```python
from build123d import *

# Parameters (mm, degrees)
SKETCH1_R           = 20
BOSS_EXTRUDE1_DEPTH = 32
SKETCH2_R           = 3
CUT_EXTRUDE1_DEPTH  = 32
CUT_EXTRUDE2_START  = -10
SKETCH3_R           = 20
SKETCH3_R_2         = 7.5
CUT_EXTRUDE2_DEPTH  = 10
SKETCH4_R           = 20
SKETCH4_R_2         = 7.5
CUT_EXTRUDE3_DEPTH  = 10
CUT_EXTRUDE4_START  = -7
SKETCH6_W           = 2
SKETCH6_H           = 4.833484819
CUT_EXTRUDE4_DEPTH  = 2


with BuildPart() as part:
    # Sketch1 → Boss-Extrude1 (new body)
    with BuildSketch(Plane.XY):
        Circle(SKETCH1_R)
    extrude(amount=BOSS_EXTRUDE1_DEPTH)

    # Sketch2 → Cut-Extrude1 (cut)
    with BuildSketch(Plane.XY.offset(32)):
        Circle(SKETCH2_R)
    extrude(amount=-CUT_EXTRUDE1_DEPTH, mode=Mode.SUBTRACT)

    # Sketch3 → Cut-Extrude2 (cut)
    with BuildSketch(Plane.XY.offset(32).offset(CUT_EXTRUDE2_START)):
        Circle(SKETCH3_R)
        Circle(SKETCH3_R_2, mode=Mode.SUBTRACT)
    extrude(amount=CUT_EXTRUDE2_DEPTH, mode=Mode.SUBTRACT)

    # Sketch4 → Cut-Extrude3 (cut)
    with BuildSketch(Plane(origin=(0, 0, 0), x_dir=(-1, 0, 0), z_dir=(0, 0, -1))):
        Circle(SKETCH4_R)
        with Locations(Location((0, 0, 0), (0, 0, 180))):
            Circle(SKETCH4_R_2, mode=Mode.SUBTRACT)
    extrude(amount=-CUT_EXTRUDE3_DEPTH, mode=Mode.SUBTRACT)

    # Sketch6 → Cut-Extrude4 (cut)
    with BuildSketch(Plane.XY.offset(32).offset(CUT_EXTRUDE4_START)):
        with Locations((0.206120499, 4.959454821)):
            Rectangle(SKETCH6_W, SKETCH6_H)
    extrude(amount=-CUT_EXTRUDE4_DEPTH, mode=Mode.SUBTRACT)


solid = part.part
```
Source: CAD feature listing. Evaluate the final solid. Frame: model axes, mm. A direction names the side the tool comes from. Coordinates: 2 decimals unless noted, no trailing zeros. Loops run counter-clockwise (first coordinate to the right, second up) from the corner with the lowest first, then second, coordinate; pieces in that order, holes last. Notation, with made-up numbers: M -32,66 L -11,66 A28 ccw -11,100 Z; hole C 81.25,-40 d4. An arc over 180 degrees is marked long. Put each result on its own line as item: value. Start each with the question number.
1) Reachability of faces 1 (the face through (4.032, -6.324, 4.93)), 2 (the face through (0, 5, 23)), 3 (the face through (-7.493, 0.33, 26.93)) from +Z, -Z, +X, -X, +Y, -Y: full face, straight path, thin tool, end or side. Return the list, or none.
2) Cut plane B-B on y = 0. Return the cut outline in (x, z).
3) Contact query for flat-ended pins moving along their axis: pin 1 Ø1 at (x, y) = (14, 9.5) entering from +Z; pin 2 Ø2 at (y, z) = (5.5, 24) entering from -X; pin 3 Ø12 at (x, z) = (-4.5, 6) entering from -Y; pin 4 Ø3.5 at (x, y) = (0, 0) entering from -Z. Output: stop coordinate, or through.
4) Pull-direction query (X, two-part tool) for faces 4 (the face through (1.206, 5, 24)), 5 (the face through (-9, 0, 10)), 6 (the face through (-4.336, -19.524, 15.916)); classes: pulls with the +X half, pulls with the -X half, needs draft (parallel to the pull), parting line crosses it, or undercut.
5) Cut plane D-D on x = -16. Return the cut outline in (y, z), then the cut area to 3 significant figures.
6) Cut plane C-C on z = 7. Return the cut outline in (x, y), then the cut area to 3 significant figures.
7) Ray query, L1, parallel to Y at x = 0, z = 17; L2, parallel to Y at x = 0, z = 9; L3, parallel to Z at x = 18, y = 5.5. Return the intervals inside material, ascending. Write a range as from..to.
8) Cut plane A-A on x = 0. Return the cut outline in (y, z).
The answers:
1. face 1: -Z
1. face 2: none
1. face 3: +Z
2. outline: M -20,10 L -7.5,10 L -7.5,0 L -3,0 L -3,32 L -7.5,32 L -7.5,22 L -20,22 Z; M 3,0 L 7.5,0 L 7.5,10 L 20,10 L 20,22 L 7.5,22 L 7.5,32 L 3,32 Z
3. pin 1: stops at z = 22
3. pin 2: stops at x = -6
3. pin 3: stops at y = -20
3. pin 4: passes through
4. face 4: undercut
4. face 5: needs draft
4. face 6: parting line crosses it
5. outline: M -12,10 L 12,10 L 12,22 L -12,22 Z
5. area: 288 mm²
6. outline: C 0,0 d15; hole C 0,0 d6
6. area: 148 mm²
7. L1: y = -20..-3, 3..20
7. L2: y = -7.5..-3, 3..7.5
7. L3: z = 10..22
8. outline: M -20,10 L -7.5,10 L -7.5,0 L -3,0 L -3,32 L -7.5,32 L -7.5,22 L -20,22 Z; M 3,0 L 7.5,0 L 7.5,10 L 20,10 L 20,22 L 7.5,22 L 7.5,32 L 3,32 L 3,25 L 7.38,25 L 7.38,23 L 3,23 Z
